Source: CAD feature listing. Evaluate the final solid. Frame: model axes, mm. A direction names the side the tool comes from. Give positions to 0.01 mm unless a question says otherwise; leave off trailing zeros. Order: outer loops, then holes, each group sorted by start corner. A loop starts at its lowest first (then second) coordinate and runs counter-clockwise, first axis right, second up.
```python
from build123d import *

# Parameters (mm, degrees)
F0_R     = 12.5
F1_DEPTH = 21.5
F2_R     = 0.5


with BuildPart() as f1:
    # F0 (on Right) → F1 (new body)
    with BuildSketch(Plane.YZ):
        Circle(F0_R)
        with BuildLine():
            ThreePointArc((-11.189467, 2.654396), (-10.93715, 3.553695), (-10.612684, 4.429553))
            ThreePointArc((-10.612684, 4.429553), (-4.349611, 5.986726), (-0.933255, 11.462069))
            ThreePointArc((-0.933255, 11.462069), (0, 11.5), (0.933255, 11.462069))
            ThreePointArc((0.933255, 11.462069), (4.349611, 5.986726), (10.612684, 4.429553))
            ThreePointArc((10.612684, 4.429553), (10.93715, 3.553695), (11.189467, 2.654396))
            ThreePointArc((11.189467, 2.654396), (7.037818, -2.286726), (7.492255, -8.724455))
            ThreePointArc((7.492255, -8.724455), (6.75953, -9.303695), (5.982216, -9.821562))
            ThreePointArc((5.982216, -9.821562), (0, -7.4), (-5.982216, -9.821562))
            ThreePointArc((-5.982216, -9.821562), (-6.75953, -9.303695), (-7.492255, -8.724455))
            ThreePointArc((-7.492255, -8.724455), (-7.037818, -2.286726), (-11.189467, 2.654396))
        make_face(mode=Mode.SUBTRACT)
    extrude(amount=F1_DEPTH)

    # F2
    f2_edges = [f1.edges().sort_by_distance(p)[0] for p in [
        (10.75, -0.933255, 11.462069),
        (10.75, 0.933255, 11.462069),
        (10.75, -10.612684, 4.429553),
        (10.75, -11.189467, 2.654396),
        (10.75, -7.492255, -8.724455),
        (10.75, -5.982216, -9.821562),
        (10.75, 5.982216, -9.821562),
        (10.75, 11.189467, 2.654396),
    ]]
    fillet(f2_edges, radius=F2_R)


solid = f1.part
```
1) Draft query along Z for faces 1 (the flat face through (0, 0, -8)), 2 (the cylindrical face through (10.599, 11.923, 3.755)), 3 (the cylindrical face through (10.6, 4.43, 5.93)). Return one class per face: +Z half, -Z half, draft (parallel to the pull), parting line (faces both ways), or undercut.
Report:
face 1: draft
face 2: parting line
face 3: undercut
2) Material intervals for L1, parallel to Y at x = 18.5, z = -5.25; L2, parallel to Z at x = 4.25, y = 0.5; L3, parallel to Y at x = 11.25, z = 10, sorted ascending.
Report:
L1: y = -11.34 to -6.62, 6.62 to 11.34
L2: z = -12.49 to -7.41, 11.49 to 12.49
L3: y = -7.5 to -1.32, 1.32 to 7.5
3) Section query A-A, the plane y = 0. Return the cut outline in (x, z), and give its area (3 significant figures).
Report:
outline: (0, -12.5) - (21.5, -12.5) - (21.5, -7.4) - (0, -7.4) - close; (0, 11.5) - (21.5, 11.5) - (21.5, 12.5) - (0, 12.5) - close
area: 131 mm2
4) Section query B-B, the plane z = 2. Return the cut outline in (x, y).
Report:
outline: (0, -12.34) - (21.5, -12.34) - (21.5, -10.14) - (0, -10.14) - close; (0, 10.14) - (21.5, 10.14) - (21.5, 12.34) - (0, 12.34) - close
5) Pin query (flat end, axial travel): pin 1 (3 mm diameter, centred on x = 15, z = -8.5, fed in from -Y); pin 2 (12 mm diameter, centred on y = -4, z = 1, fed in from -X); pin 3 (12 mm diameter, centred on x = 11, y = 8, fed in from -Z); pin 4 (3 mm diameter, centred on x = 16.5, y = -8.5, fed in from -Z). Return the tip coordinate at first contact, or that it passes through.
Report:
pin 1: stops at y = -10.36
pin 2: stops at x = 0
pin 3: stops at z = -12.34
pin 4: stops at z = -10.36
6) Reachability of faces 4 (the cylindrical face through (10.6, -7, -2.4)), 5 (the flat face through (21.5, 0, -8)) from +Z, -Z, +X, -X, +Y, -Y: full face, straight path, thin tool, end or side. Return the list, or none.
Report:
face 4: +X, -X
face 5: +Z, -Z, +X, +Y, -Y
